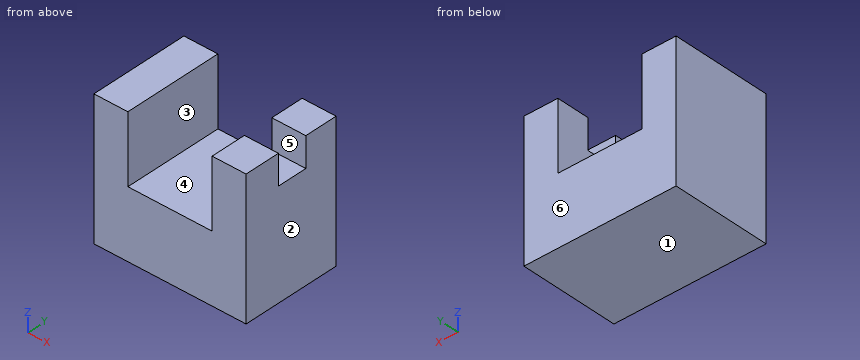
```python
from build123d import *

# Parameters (mm, degrees)
F1_DEPTH = 25.4
F2_DEPTH = 19.304
F3_W     = 15.2846500278
F3_H     = 13.6232702062
F4_DEPTH = 13.462


with BuildPart() as f1:
    # F0 (on Front) → F1 (new body)
    with BuildSketch(Plane.XZ):
        Polygon((0, 61.4708550274), (0, 0), (68.4486366808, 0), (68.4486366808, 61.4708550274), (53.1639866531, 61.4708550274), (53.1639866531, 30.7354275137), (15.2846500278, 30.7354275137), (15.2846500278, 61.4708550274), align=None)
    extrude(amount=F1_DEPTH)

    # F2 (add): a face of the model
    f2_faces = [f1.faces().sort_by_distance(p)[0] for p in [
        (34.2243183404, -25.4, 24.8565047474),
    ]]
    extrude(f2_faces, amount=F2_DEPTH)

    # F3 (on face) → F4 (cut)
    with BuildSketch(Plane.XY.offset(61.4708550274)):
        with Locations((60.806311667, -21.8535889871)):
            Rectangle(F3_W, F3_H)
    extrude(amount=-F4_DEPTH, mode=Mode.SUBTRACT)


solid = f1.part
```
For this review, take the finished solid that the model builds, in its own axes (mm). Face numbers are marked on the shaded views. A direction names the side the tool comes from. Coordinates: 2 decimals unless noted, no trailing zeros. Write each loop counter-clockwise with the first axis right and the second up, starting at its lowest first coordinate (ties: lowest second). Pieces come first, ordered by that corner, then holes.
(1) For pin 1 Ø7 at (x, y) = (57.5, -22) entering from +Z, flat-tipped, find the tip position at first contact; note if it passes through.
(2) Wall thickness on probe 1 along X at (y, z) = (-32, 57.5); probe 2 along Z at (x, y) = (55.5, -17.5); probe 3 along Z at (x, y) = (30, -6): over which ranges is each line inside the solid? List them lowest first.
(3) Add section C-C on y = -16.5. Give the boundary of the cut face in (x, z), then the cut area to 3 significant figures.
(4) The part is to be moulded in two halves that separate along X. For the marked faces 1, 2 and 3, say which applies: +X half, -X half, draft (parallel to the pull), parting line (faces both ways), or undercut.
(5) Add section B-B on z = 50. Give the boundary of the cut face in (x, y).
(6) Tool access review of the marked faces 4, 5 and 6: name each direction out of +Z, -Z, +X, -X, +Y, -Y from which nothing blocks a thin tool from reaching the whole face with its end or side.
(7) Add section A-A on z = 33. Give the boundary of the cut face in (x, y).
(8) Add section D-D on x = 56.5. Give the boundary of the cut face in (y, z), then the cut area to 3 significant figures.
Answer sheet:
1. pin 1: stops at z = 48.01
2. probe 1: x = 0 to 15.28, 53.16 to 68.45
2. probe 2: z = 0 to 48.01
2. probe 3: z = 0 to 30.74
3. outline: (0, 0) - (68.45, 0) - (68.45, 48.01) - (53.16, 48.01) - (53.16, 30.74) - (15.28, 30.74) - (15.28, 61.47) - (0, 61.47) - close
3. area: 2,840 mm2
4. face 1: draft
4. face 2: +X half
4. face 3: undercut
5. outline: (0, -44.7) - (15.28, -44.7) - (15.28, 0) - (0, 0) - close; (53.16, -44.7) - (68.45, -44.7) - (68.45, -28.67) - (53.16, -28.67) - close; (53.16, -15.04) - (68.45, -15.04) - (68.45, 0) - (53.16, 0) - close
6. face 4: +Z, +Y, -Y
6. face 5: +Z, +X
6. face 6: +Z, -Z, +X, -X, +Y
7. outline: (0, -44.7) - (15.28, -44.7) - (15.28, 0) - (0, 0) - close; (53.16, -44.7) - (68.45, -44.7) - (68.45, 0) - (53.16, 0) - close
8. outline: (-44.7, 0) - (0, 0) - (0, 61.47) - (-15.04, 61.47) - (-15.04, 48.01) - (-28.67, 48.01) - (-28.67, 61.47) - (-44.7, 61.47) - close
8. area: 2,560 mm2
